Geometry check sheet. Reference: the model listing, model coordinates, mm. A direction names the side the tool comes from. Coordinates: 2 decimals unless noted, no trailing zeros. Write each loop counter-clockwise with the first axis right and the second up, starting at its lowest first coordinate (ties: lowest second). Pieces come first, ordered by that corner, then holes. Notation, with made-up numbers: M 87,58 L 128,58 A19 ccw 128,63 Z; hole C 29,28.5 d6. An arc over 180 degrees is marked long. Answer as a JSON object with one key per item and string values. Group by question number.
```python
from build123d import *

# Parameters (mm, degrees)
RESSALTO_EXTRUS_O1_DEPTH                            = 3
ESBO_O2_W                                           = 50
ESBO_O2_H                                           = 105
RESSALTO_EXTRUS_O2_DEPTH                            = 3
RESSALTO_EXTRUS_O3_DEPTH                            = 3
REBAIXO_PARA_SHCS_M21_D                             = 2.4
REBAIXO_PARA_SHCS_M21_DEPTH                         = 3
REBAIXO_PARA_SHCS_M21_CBORE_D                       = 4.4
REBAIXO_PARA_SHCS_M21_CBORE_DEPTH                   = 2
PADR_OCIRCULAR1_COUNT                               = 5
PADR_OCIRCULAR1_ANGLE                               = 180
NERVURA1_REACH                                      = 104.147
ESBO_O6_WALL_W                                      = 216.193400866
ESBO_O6_WALL_H                                      = 15
CORTE_EXTRUS_O1_REACH                               = 106.943
ESBO_O7_W                                           = 10
ESBO_O7_H                                           = 7
NERVURA7_REACH                                      = 104.147
ESBO_O8_WALL_W                                      = 216.193400866
ESBO_O8_WALL_H                                      = 15
CORTE_EXTRUS_O2_REACH                               = 104.147
ESBO_O9_W                                           = 10
ESBO_O9_H                                           = 7
PADR_O_LINEAR1_COUNT                                = 2
PADR_O_LINEAR1_PITCH                                = 84.45
ESBO_O10_R                                          = 2.75
RESSALTO_EXTRUS_O4_DEPTH                            = 0.6
REBAIXO_PARA_PARAFUSO_COM_CABE_A_PANELA_D           = 3.4
REBAIXO_PARA_PARAFUSO_COM_CABE_A_PANELA_CBORE_D     = 7
REBAIXO_PARA_PARAFUSO_COM_CABE_A_PANELA_CBORE_DEPTH = 1.5
FILETE1_R                                           = 5


with BuildPart() as part:
    # Esboço1 → Ressalto-extrusão1 (new body)
    with BuildSketch(Plane.XY):
        with BuildLine():
            Line((11, 0), (11, 25))
            Line((11, 25), (-11, 25))
            Line((-11, 25), (-11, 0))
            ThreePointArc((-11, 0), (-7.75, -3.25), (-4.5, 0))
            ThreePointArc((-4.5, 0), (0, 4.5), (4.5, 0))
            ThreePointArc((4.5, 0), (7.75, -3.25), (11, 0))
        make_face()
    extrude(amount=RESSALTO_EXTRUS_O1_DEPTH)

    # Esboço2 → Ressalto-extrusão2 (add)
    with BuildSketch(Plane(origin=(0, 25, 0), x_dir=(1, 0, 0), z_dir=(0, 1, 0))):
        with Locations((0, 42.5)):
            Rectangle(ESBO_O2_W, ESBO_O2_H)
    extrude(amount=RESSALTO_EXTRUS_O2_DEPTH)

    # Esboço3 → Ressalto-extrusão3 (add)
    with BuildSketch(Plane(origin=(0, 0, -81.45), x_dir=(-1, 0, 0), z_dir=(0, 0, -1))):
        with BuildLine():
            Line((-11, 0), (-11, 25))
            Line((-11, 25), (11, 25))
            Line((11, 25), (11, 0))
            ThreePointArc((11, 0), (0, -11), (-11, 0))
        make_face()
    extrude(amount=RESSALTO_EXTRUS_O3_DEPTH)

    # Rebaixo para SHCS M21
    with Locations(Plane.XY.offset(3)):
        with Locations((8, 0)):
            rebaixo_para_shcs_m21 = CounterBoreHole(REBAIXO_PARA_SHCS_M21_D / 2, REBAIXO_PARA_SHCS_M21_CBORE_D / 2, REBAIXO_PARA_SHCS_M21_CBORE_DEPTH, depth=REBAIXO_PARA_SHCS_M21_DEPTH)

    # PadrãoCircular1: Rebaixo para SHCS M21 ×5 about axis
    padr_ocircular1_axis = Axis((0, 0, 0), (0, 0, 1))
    for i in range(1, PADR_OCIRCULAR1_COUNT):
        add(rebaixo_para_shcs_m21.rotate(padr_ocircular1_axis, i * PADR_OCIRCULAR1_ANGLE / (PADR_OCIRCULAR1_COUNT - 1)), mode=Mode.SUBTRACT)

    # Esboço6 wall → Nervura1 (add, up to next)
    with BuildSketch(Plane(origin=(0, 21.5, 6.5), x_dir=(0, 0.707106781187, 0.707106781187), z_dir=(0, -0.707106781187, 0.707106781187)), mode=Mode.PRIVATE) as nervura1_sk1:
        Rectangle(ESBO_O6_WALL_W, ESBO_O6_WALL_H)
    nervura1_tool1 = extrude(nervura1_sk1.sketch, amount=-NERVURA1_REACH, mode=Mode.PRIVATE) - part.part
    nervura1 = nervura1_tool1.solids().sort_by_distance((0, 21.5, 6.5))[0]
    add(nervura1)

    # Corte-extrusão1: up to this face of the body (flat: up to its plane)
    corte_extrus_o1_end = Plane(part.part.faces().sort_by_distance((0, 21.5, 6.5))[0])
    # Esboço7 → Corte-extrusão1 (cut, up to the picked face)
    with BuildSketch(Plane.XY.offset(3), mode=Mode.PRIVATE) as corte_extrus_o1_sk1:
        with Locations((0, 21.5)):
            Rectangle(ESBO_O7_W, ESBO_O7_H)
    corte_extrus_o1_tool1 = split(extrude(corte_extrus_o1_sk1.sketch, amount=CORTE_EXTRUS_O1_REACH, mode=Mode.PRIVATE), bisect_by=corte_extrus_o1_end, keep=Keep.BOTH, mode=Mode.PRIVATE)
    corte_extrus_o1 = corte_extrus_o1_tool1.solids().sort_by(Axis((0, 21.5, 3), (0, 0, 1)))[0]
    add(corte_extrus_o1, mode=Mode.SUBTRACT)

    # Esboço8 wall → Nervura7 (add, up to next)
    with BuildSketch(Plane(origin=(0, 21.5, -3.5), x_dir=(0, 0.707106781187, -0.707106781187), z_dir=(0, 0.707106781187, 0.707106781187)), mode=Mode.PRIVATE) as nervura7_sk1:
        Rectangle(ESBO_O8_WALL_W, ESBO_O8_WALL_H)
    nervura7_tool1 = extrude(nervura7_sk1.sketch, amount=NERVURA7_REACH, mode=Mode.PRIVATE) - part.part
    nervura7 = nervura7_tool1.solids().sort_by_distance((0, 21.5, -3.5))[0]
    add(nervura7)

    # Corte-extrusão2: up to this face of the body (flat: up to its plane)
    corte_extrus_o2_end = Plane(part.part.faces().sort_by_distance((0, 21.5, -3.5))[0])
    # Esboço9 → Corte-extrusão2 (cut, up to the picked face)
    with BuildSketch(Plane(origin=(0, 0, 0), x_dir=(-1, 0, 0), z_dir=(0, 0, -1)), mode=Mode.PRIVATE) as corte_extrus_o2_sk1:
        with Locations((0, 21.5)):
            Rectangle(ESBO_O9_W, ESBO_O9_H)
    corte_extrus_o2_tool1 = split(extrude(corte_extrus_o2_sk1.sketch, amount=CORTE_EXTRUS_O2_REACH, mode=Mode.PRIVATE), bisect_by=corte_extrus_o2_end, keep=Keep.BOTH, mode=Mode.PRIVATE)
    corte_extrus_o2 = corte_extrus_o2_tool1.solids().sort_by(Axis((0, 21.5, 0), (0, 0, -1)))[0]
    add(corte_extrus_o2, mode=Mode.SUBTRACT)

    # Padrão linear1: Nervura1, Corte-extrusão1, Nervura7, Corte-extrusão2 ×2
    with Locations(*[(0, 0, -i * PADR_O_LINEAR1_PITCH) for i in range(1, PADR_O_LINEAR1_COUNT)]):
        add(nervura1)
        add(corte_extrus_o1, mode=Mode.SUBTRACT)
        add(nervura7)
        add(corte_extrus_o2, mode=Mode.SUBTRACT)

    # Esboço10 → Ressalto-extrusão4 (add)
    with BuildSketch(Plane.XY.offset(-81.45)):
        with Locations(Location((0, 0, 0), (0, 0, 180))):
            Circle(ESBO_O10_R)
    extrude(amount=RESSALTO_EXTRUS_O4_DEPTH)

    # Rebaixo para parafuso com cabeça panela de M31 (through all)
    with Locations(Plane(origin=(0, 0, -84.45), x_dir=(-1, 0, 0), z_dir=(0, 0, -1))):
        with Locations((0, 0)):
            CounterBoreHole(REBAIXO_PARA_PARAFUSO_COM_CABE_A_PANELA_D / 2, REBAIXO_PARA_PARAFUSO_COM_CABE_A_PANELA_CBORE_D / 2, REBAIXO_PARA_PARAFUSO_COM_CABE_A_PANELA_CBORE_DEPTH)

    # Filete1
    filete1_edges = [part.edges().sort_by_distance(p)[0] for p in [
        (-11, 25, 1.5),
        (11, 25, 1.5),
        (0, 25, 3),
        (9.25, 25, 3),
        (-9.25, 25, 0),
        (0, 25, 0),
        (9.25, 25, -81.45),
        (0, 25, -81.45),
        (9.25, 25, -84.45),
        (0, 25, -84.45),
        (-9.25, 25, -81.45),
        (-11, 25, -82.95),
        (11, 25, -82.95),
        (-9.25, 25, -84.45),
        (9.25, 25, 0),
        (-9.25, 25, 3),
    ]]
    fillet(filete1_edges, radius=FILETE1_R)


solid = part.part
```
1) Section check D-D (x = 0). State how many separate pieces and enclosed holes the cut face has, then the cut area to 3 significant figures.
2) Material ranges on probe 1 along Z at (x, y) = (9, 4.5); probe 2 along Y at (x, z) = (-8, 2.6); probe 3 along Y at (x, z) = (8, 0.6), recorded low to high. Write a range as [from, to].
3) Draft check along Y on faces 4 (the cylindrical face through (-10.87, 24.13, -86.63)), 5 (the flat face through (5, 22, -87)), 6 (the cylindrical face through (0.596, 2.685, -81.154)), 7 (the cylindrical face through (6.847, 5.814, 0.493)). Enter one of: +Y half, -Y half, draft (parallel to the pull), parting line (faces both ways), or undercut.
4) Section check C-C (x = -15). Record the cut outline in (y, z), then the cut area to 3 significant figures.
5) Section check A-A (y = 11.5). Record the cut outline in (x, z).
6) Section check B-B (z = -88). Record the cut outline in (x, y), then the cut area to 3 significant figures.
7) Set-up check for faces 1 (the cylindrical face through (-3.233, -1.341, -83.71)), 2 (the flat face through (-7.5, 22, -3)), 3 (the cylindrical face through (9.2, 0.05, 0.49)): record each of +Z, -Z, +X, -X, +Y, -Y from which the full face is reachable in a straight line by a thin tool's end or side.
8) Go/stop test with flat-tipped pins: pin 1 Ø2 at (y, z) = (22, -77) entering from +X; pin 2 Ø2 at (x, y) = (-1, -0.5) entering from -Z; pin 3 Ø1 at (x, z) = (-5, -5) entering from -Y. Record where each tip stops, or that it passes through.
Entries:
{
 "1": {"separate pieces": "3", "enclosed holes": "0", "area": "480 mm^2"},
 "2": {"probe 1": "[-84.45, -81.45], [0, 3]", "probe 2": "[-3.24, -2.2], [2.2, 28]", "probe 3": "[-3.24, -1.2], [1.2, 28]"},
 "3": {"face 4": "-Y half", "face 5": "draft", "face 6": "undercut", "face 7": "undercut"},
 "4": {"outline": "M 24.9,-88.45 A5 cw 25,-89.45 L 25,-95 L 28,-95 L 28,10 L 25,10 L 25,8 A5 cw 24.9,7 L 24.9,-4 A5 cw 25,-5 L 25,-76.45 A5 cw 24.9,-77.45 Z", "area": "317 mm^2"},
 "5": {"outline": "M -11,-84.45 L 11,-84.45 L 11,-81.45 L -11,-81.45 Z; M -11,0 L 11,0 L 11,3 L -11,3 Z"},
 "6": {"outline": "M -25,25 L -16,25 A5 cw -14.55,24.79 L -7.5,24.79 L -7.5,21.55 L -5,21.55 L -5,24.79 L 5,24.79 L 5,21.55 L 7.5,21.55 L 7.5,24.79 L 14.55,24.79 A5 cw 16,25 L 25,25 L 25,28 L -25,28 Z", "area": "173 mm^2"},
 "7": {"face 1": "-Z", "face 2": "-X, -Y", "face 3": "+Z"},
 "8": {"pin 1": "x = 7.5", "pin 2": "z = -82.95", "pin 3": "y = 22.5"}
}
